Part model, mm, in its own coordinate system. Round coordinates to 2 decimals unless told otherwise and drop trailing zeros. Order: outer loops, then holes, each group sorted by start corner. A loop starts at its lowest first (then second) coordinate and runs counter-clockwise, first axis right, second up. Notation, with made-up numbers: M 54.25,-19 L 83.25,-19 A10 ccw 83.25,-15 Z; hole C 64.25,88 d6. An arc over 180 degrees is marked long. One line per question, with ' | ' between items.
from build123d import *

# Parameters (mm, degrees)
F0_R     = 1.65
F1_DEPTH = 1.5
F2_R     = 1


with BuildPart() as f1:
    # F0 (on Front) → F1 (new body)
    with BuildSketch(Plane.XZ):
        Polygon((0, 15), (-50, 15), (-50, -15), (0, -15), (50, -15), (50, 15), align=None)
        with Locations((-45, 0)):
            Circle(F0_R, mode=Mode.SUBTRACT)
        with Locations((45, 0)):
            Circle(F0_R, mode=Mode.SUBTRACT)
    extrude(amount=F1_DEPTH)

    # F2
    f2_edges = [f1.edges().sort_by_distance(p)[0] for p in [
        (50, -0.75, 15),
        (50, -0.75, -15),
        (-50, -0.75, 15),
        (-50, -0.75, -15),
    ]]
    fillet(f2_edges, radius=F2_R)


solid = f1.part
1) Saw through at B-B (x = 45). List the corners of the cut face in (y, z), plus the area to 4 significant figures.
The answers:
outline: M -1.5,-15 L 0,-15 L 0,-1.65 L -1.5,-1.65 Z; M -1.5,1.65 L 0,1.65 L 0,15 L -1.5,15 Z | area: 40.05 mm²
2) Saw through at A-A (z = 0). List the corners of the cut face in (x, y).
The answers:
outline: M -50,-1.5 L -46.65,-1.5 L -46.65,0 L -50,0 Z; M -43.35,-1.5 L 43.35,-1.5 L 43.35,0 L -43.35,0 Z; M 46.65,-1.5 L 50,-1.5 L 50,0 L 46.65,0 Z
3) Probe line 1 (X direction, y = -0.2, z = 0.75); line 2 (Z direction, x = -45, y = -0.7); line 3 (Z direction, x = -44, y = -0.7). List the from-to ranges inside material, lowest first. Write a range as [from, to].
The answers:
line 1: x = [-50, -46.47], [-43.53, 43.53], [46.47, 50] | line 2: z = [-15, -1.65], [1.65, 15] | line 3: z = [-15, -1.31], [1.31, 15]
4) Two-plate mould, pull along X, no slides. Class faces 1 (the face through (43.35, -0.74, 0.07)), 2 (the face through (-1, -1.5, 0)): released by +X, released by -X, zero draft, split by the parting line, or undercut.
The answers:
face 1: undercut | face 2: zero draft
